Check sheet for the modelled part. Datum: model origin and axes. Units: mm. Face numbers are marked on the shaded views. A direction names the side the tool comes from. Round coordinates to 2 decimals unless told otherwise and drop trailing zeros. Loops run counter-clockwise (first coordinate to the right, second up) from the corner with the lowest first, then second, coordinate; pieces in that order, holes last. Notation, with made-up numbers: M 7,1 L 11,1 A24 cw 11,13 Z; hole C 24.5,-34 d2. An arc over 180 degrees is marked long. One line per question, with ' | ' between items. Start each with the question number.
(1) Section check D-D (z = 17.95). Record the boundary of the cut face in (x, y).
(2) Thickness scan on probe 1 along Z at (x, y) = (0, 0.7); probe 2 along X at (y, z) = (0.7, 3); probe 3 along Z at (x, y) = (17.95, -0.8). Record the ranges inside material, lowest first. Write a range as [from, to].
(3) Section check B-B (z = 3.5). Record the boundary of the cut face in (x, y), and give its area (3 significant figures).
(4) Section check C-C (y = -0.95). Record the boundary of the cut face in (x, z), and give its area (3 significant figures).
(5) Go/stop test with flat-tipped pins: P1, Ø1.2, axis at x = 13.5, y = -0.5, coming from the +Z side; P2, Ø1.2, axis at x = 0, z = 17.95, coming from the +Y side; P3, Ø2, axis at y = 0, z = 12, coming from the -X side; P4, Ø2, axis at x = -13, y = 0, coming from the +Z side. Record where each tip stops, or that it passes through.
(6) Section check A-A (x = 0). Record the boundary of the cut face in (y, z), and give its area (3 significant figures).
(7) Draft check along X on the marked faces 3, 4 and 5. Enter one of: +X half, -X half, draft (parallel to the pull), parting line (faces both ways), or undercut.
(8) Tool access check on the marked faces 1 and 2. Record the directions out of +Z, -Z, +X, -X, +Y, -Y that give a thin tool (end or side, any length) a straight path to the whole face; none if there is none.
```python
from build123d import *

# Parameters (mm, degrees)
CROQUIS1_W                 = 39.9
CROQUIS1_H                 = 39.9
SALIENTE_EXTRUIR1_DEPTH    = 2
CROQUIS7_W                 = 4
CROQUIS7_H                 = 20
CORTAR_EXTRUIR3_DEPTH      = 3
CORTAR_EXTRUIR3_DEPTH_BACK = 3
CROQUIS9_R                 = 1
CORTAR_EXTRUIR4_DEPTH      = 1
CORTAR_EXTRUIR4_DEPTH_BACK = 5
REDONDEO8_R                = 3
CROQUIS10_W                = 9.5
CROQUIS10_H                = 20.95
CORTAR_EXTRUIR5_DEPTH      = 1
CORTAR_EXTRUIR5_DEPTH_BACK = 5


with BuildPart() as part:
    # Croquis1 → Saliente-Extruir1 (new body, symmetric)
    with BuildSketch(Plane(origin=(0, 0, 0), x_dir=(1, 0, 0), z_dir=(0, 1, 0))):
        Rectangle(CROQUIS1_W, CROQUIS1_H)
    extrude(amount=SALIENTE_EXTRUIR1_DEPTH, both=True)

    # Croquis7 → Cortar-Extruir3 (cut, two sides)
    with BuildSketch(Plane(origin=(0, 0, 0), x_dir=(1, 0, 0), z_dir=(0, 1, 0))) as cortar_extruir3_sk:
        with Locations((13.95, -9.95)):
            Rectangle(CROQUIS7_W, CROQUIS7_H)
        with Locations((-13.95, -9.95)):
            Rectangle(CROQUIS7_W, CROQUIS7_H)
    extrude(amount=CORTAR_EXTRUIR3_DEPTH, mode=Mode.SUBTRACT)
    extrude(cortar_extruir3_sk.sketch, amount=-CORTAR_EXTRUIR3_DEPTH_BACK, mode=Mode.SUBTRACT)

    # Croquis9 → Cortar-Extruir4 (cut, two sides)
    with BuildSketch(Plane.XZ.offset(2)) as cortar_extruir4_sk:
        with Locations((0, 17.95)):
            Circle(CROQUIS9_R)
        with Locations((-17.95, 0)):
            Circle(CROQUIS9_R)
        with Locations((0, -17.95)):
            Circle(CROQUIS9_R)
        with Locations((17.95, 0)):
            Circle(CROQUIS9_R)
    extrude(amount=CORTAR_EXTRUIR4_DEPTH, mode=Mode.SUBTRACT)
    extrude(cortar_extruir4_sk.sketch, amount=-CORTAR_EXTRUIR4_DEPTH_BACK, mode=Mode.SUBTRACT)

    # Redondeo8
    redondeo8_edges = [part.edges().sort_by_distance(p)[0] for p in [
        (19.95, 0, 19.95),
        (-19.95, 0, 19.95),
        (-19.95, 0, -19.95),
        (19.95, 0, -19.95),
    ]]
    fillet(redondeo8_edges, radius=REDONDEO8_R)

    # Croquis10 → Cortar-Extruir5 (cut, two sides)
    with BuildSketch(Plane(origin=(0, 2, 0), x_dir=(1, 0, 0), z_dir=(0, 1, 0))) as cortar_extruir5_sk:
        with Locations((-15.2, -9.475)):
            Rectangle(CROQUIS10_W, CROQUIS10_H)
    extrude(amount=CORTAR_EXTRUIR5_DEPTH, mode=Mode.SUBTRACT)
    extrude(cortar_extruir5_sk.sketch, amount=-CORTAR_EXTRUIR5_DEPTH_BACK, mode=Mode.SUBTRACT)


solid = part.part
```
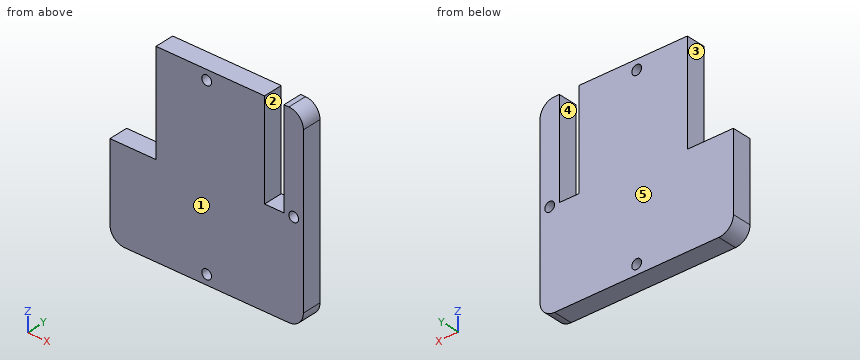
The answers:
1) outline: M -10.45,-2 L -1,-2 L -1,2 L -10.45,2 Z; M 1,-2 L 11.95,-2 L 11.95,2 L 1,2 Z; M 15.95,-2 L 19.78,-2 L 19.78,2 L 15.95,2 Z
2) probe 1: [-19.95, -18.95], [-16.95, 16.95], [18.95, 19.95] | probe 2: [-10.45, 11.95], [15.95, 19.95] | probe 3: [-19.78, -1], [1, 19.78]
3) outline: M -10.45,-2 L 11.95,-2 L 11.95,2 L -10.45,2 Z; M 15.95,-2 L 19.95,-2 L 19.95,2 L 15.95,2 Z | area: 106 mm²
4) outline: M -19.95,-16.95 A3 ccw -16.95,-19.95 L 16.95,-19.95 A3 ccw 19.95,-16.95 L 19.95,16.95 A3 ccw 16.95,19.95 L 15.95,19.95 L 15.95,-0.05 L 11.95,-0.05 L 11.95,19.95 L -10.45,19.95 L -10.45,-1 L -19.95,-1 Z; hole C 0,-17.95 d2; hole C 0,17.95 d2; hole C 17.95,0 d2 | area: 1,300 mm²
5) P1: z = -0.05 | P2: through | P3: x = -10.45 | P4: z = -1
6) outline: M -2,-19.95 L 2,-19.95 L 2,-18.95 L -2,-18.95 Z; M -2,-16.95 L 2,-16.95 L 2,16.95 L -2,16.95 Z; M -2,18.95 L 2,18.95 L 2,19.95 L -2,19.95 Z | area: 144 mm²
7) face 3: -X half | face 4: undercut | face 5: draft
8) face 1: +Z, -Z, +X, -X, -Y | face 2: +Z, +Y, -Y
